Geometry check sheet. Reference: the model listing, model coordinates, mm. A direction names the side the tool comes from. Coordinates: 2 decimals unless noted, no trailing zeros. Order: outer loops, then holes, each group sorted by start corner. A loop starts at its lowest first (then second) coordinate and runs counter-clockwise, first axis right, second up. Notation, with made-up numbers: (1, 40) - (20, 40) arc R3 ccw to (20, 45) - close; hole circle Ø3 at (51.5, 21.25). An arc over 180 degrees is marked (long way). Put each result on its own line as item: value.
from build123d import *

# Parameters (mm, degrees)
SKETCH_1_R          = 42.5
SKETCH_1_R_2        = 35.25
EXTRUDE_1_DEPTH     = 2.5
SKETCH_2_R          = 1.5
CUT_EXTRUDE_1_DEPTH = 61.156047078
SKETCH_3_R          = 41.5
SKETCH_3_R_2        = 37.9
CUT_EXTRUDE_2_DEPTH = 0.5


with BuildPart() as part:
    # 草图1 → 凸台-拉伸1 (new body)
    with BuildSketch(Plane(origin=(0, 0, 0), x_dir=(1, 0, 0), z_dir=(0, 1, 0))):
        with Locations(Location((0, 0, 0), (0, 0, 270))):
            Circle(SKETCH_1_R)
        with Locations(Location((0, 0, 0), (0, 0, 270))):
            Circle(SKETCH_1_R_2, mode=Mode.SUBTRACT)
    extrude(amount=EXTRUDE_1_DEPTH)

    # 草图2 → 切除-拉伸1 (cut, through all)
    with BuildSketch(Plane.XZ):
        with Locations(Location((0, 40, 0), (0, 0, 270))):
            Circle(SKETCH_2_R)
        with Locations(Location((28.284271247, 28.284271247, 0), (0, 0, 270))):
            Circle(SKETCH_2_R)
        with Locations(Location((40, 0, 0), (0, 0, 270))):
            Circle(SKETCH_2_R)
        with Locations(Location((28.284271247, -28.284271247, 0), (0, 0, 270))):
            Circle(SKETCH_2_R)
        with Locations(Location((0, -40, 0), (0, 0, 270))):
            Circle(SKETCH_2_R)
        with Locations(Location((-28.284271247, -28.284271247, 0), (0, 0, 270))):
            Circle(SKETCH_2_R)
        with Locations(Location((-40, 0, 0), (0, 0, 270))):
            Circle(SKETCH_2_R)
        with Locations(Location((-28.284271247, 28.284271247, 0), (0, 0, 270))):
            Circle(SKETCH_2_R)
    extrude(amount=-CUT_EXTRUDE_1_DEPTH, mode=Mode.SUBTRACT)

    # 草图3 → 切除-拉伸2 (cut)
    with BuildSketch(Plane(origin=(0, 2.5, 0), x_dir=(1, 0, 0), z_dir=(0, 1, 0))):
        with Locations(Location((0, 0, 0), (0, 0, 270))):
            Circle(SKETCH_3_R)
        with Locations(Location((0, 0, 0), (0, 0, 270))):
            Circle(SKETCH_3_R_2, mode=Mode.SUBTRACT)
    extrude(amount=-CUT_EXTRUDE_2_DEPTH, mode=Mode.SUBTRACT)

    # 打孔尺寸(%根据十字)槽沉头木螺钉的类型1: read off the stored shape, not the designer's step
    # 打孔尺寸(%根据十字)槽沉头木螺钉的类型1: loft between two sections, ruled curve by curve
    hole_wizard_1_from = [
        Edge.make_three_point_arc((-40, 1.4, -1.5), (-38.5, 1.4, 0), (-40, 1.4, 1.5)),
        Edge.make_three_point_arc((-40, 1.4, 1.5), (-41.5, 1.4, 0), (-40, 1.4, -1.5)),
    ]
    hole_wizard_1_to = [
        Edge.make_three_point_arc((-40, -4.3e-08, -2.900000043), (-37.099999957, -4.3e-08, 0), (-40, -4.3e-08, 2.900000043)),
        Edge.make_three_point_arc((-40, -4.3e-08, 2.900000043), (-42.900000043, -4.3e-08, 0), (-40, -4.3e-08, -2.900000043)),
    ]
    hole_wizard_1 = Solid(Shell([*[Face.make_surface_from_curves(hole_wizard_1_from[k], hole_wizard_1_to[k]) for k in range(2)], Face(Wire(hole_wizard_1_from)), Face(Wire(hole_wizard_1_to))]))
    add(hole_wizard_1, mode=Mode.SUBTRACT)

    # Hole Wizard 1 2: loft between two sections, ruled curve by curve
    hole_wizard_1_2_from = [
        Edge.make_three_point_arc((-28.284271247, 1.4, -29.784271247), (-26.784271247, 1.4, -28.284271247), (-28.284271247, 1.4, -26.784271247)),
        Edge.make_three_point_arc((-28.284271247, 1.4, -26.784271247), (-29.784271247, 1.4, -28.284271247), (-28.284271247, 1.4, -29.784271247)),
    ]
    hole_wizard_1_2_to = [
        Edge.make_three_point_arc((-28.284271247, -4.3e-08, -31.18427129), (-25.384271205, -4.3e-08, -28.284271247), (-28.284271247, -4.3e-08, -25.384271205)),
        Edge.make_three_point_arc((-28.284271247, -4.3e-08, -25.384271205), (-31.18427129, -4.3e-08, -28.284271247), (-28.284271247, -4.3e-08, -31.18427129)),
    ]
    hole_wizard_1_2 = Solid(Shell([*[Face.make_surface_from_curves(hole_wizard_1_2_from[k], hole_wizard_1_2_to[k]) for k in range(2)], Face(Wire(hole_wizard_1_2_from)), Face(Wire(hole_wizard_1_2_to))]))
    add(hole_wizard_1_2, mode=Mode.SUBTRACT)

    # Hole Wizard 1 3: loft between two sections, ruled curve by curve
    hole_wizard_1_3_from = [
        Edge.make_three_point_arc((0, 1.4, -41.5), (1.5, 1.4, -40), (0, 1.4, -38.5)),
        Edge.make_three_point_arc((0, 1.4, -38.5), (-1.5, 1.4, -40), (0, 1.4, -41.5)),
    ]
    hole_wizard_1_3_to = [
        Edge.make_three_point_arc((0, -4.3e-08, -42.900000043), (2.900000043, -4.3e-08, -40), (0, -4.3e-08, -37.099999957)),
        Edge.make_three_point_arc((0, -4.3e-08, -37.099999957), (-2.900000043, -4.3e-08, -40), (0, -4.3e-08, -42.900000043)),
    ]
    hole_wizard_1_3 = Solid(Shell([*[Face.make_surface_from_curves(hole_wizard_1_3_from[k], hole_wizard_1_3_to[k]) for k in range(2)], Face(Wire(hole_wizard_1_3_from)), Face(Wire(hole_wizard_1_3_to))]))
    add(hole_wizard_1_3, mode=Mode.SUBTRACT)

    # Hole Wizard 1 4: loft between two sections, ruled curve by curve
    hole_wizard_1_4_from = [
        Edge.make_three_point_arc((28.284271247, 1.4, -29.784271247), (29.784271247, 1.4, -28.284271247), (28.284271247, 1.4, -26.784271247)),
        Edge.make_three_point_arc((28.284271247, 1.4, -26.784271247), (26.784271247, 1.4, -28.284271247), (28.284271247, 1.4, -29.784271247)),
    ]
    hole_wizard_1_4_to = [
        Edge.make_three_point_arc((28.284271247, -4.3e-08, -31.18427129), (31.18427129, -4.3e-08, -28.284271247), (28.284271247, -4.3e-08, -25.384271205)),
        Edge.make_three_point_arc((28.284271247, -4.3e-08, -25.384271205), (25.384271205, -4.3e-08, -28.284271247), (28.284271247, -4.3e-08, -31.18427129)),
    ]
    hole_wizard_1_4 = Solid(Shell([*[Face.make_surface_from_curves(hole_wizard_1_4_from[k], hole_wizard_1_4_to[k]) for k in range(2)], Face(Wire(hole_wizard_1_4_from)), Face(Wire(hole_wizard_1_4_to))]))
    add(hole_wizard_1_4, mode=Mode.SUBTRACT)

    # Hole Wizard 1 5: loft between two sections, ruled curve by curve
    hole_wizard_1_5_from = [
        Edge.make_three_point_arc((40, 1.4, -1.5), (41.5, 1.4, 0), (40, 1.4, 1.5)),
        Edge.make_three_point_arc((40, 1.4, 1.5), (38.5, 1.4, 0), (40, 1.4, -1.5)),
    ]
    hole_wizard_1_5_to = [
        Edge.make_three_point_arc((40, -4.3e-08, -2.900000043), (42.900000043, -4.3e-08, 0), (40, -4.3e-08, 2.900000043)),
        Edge.make_three_point_arc((40, -4.3e-08, 2.900000043), (37.099999957, -4.3e-08, 0), (40, -4.3e-08, -2.900000043)),
    ]
    hole_wizard_1_5 = Solid(Shell([*[Face.make_surface_from_curves(hole_wizard_1_5_from[k], hole_wizard_1_5_to[k]) for k in range(2)], Face(Wire(hole_wizard_1_5_from)), Face(Wire(hole_wizard_1_5_to))]))
    add(hole_wizard_1_5, mode=Mode.SUBTRACT)

    # Hole Wizard 1 6: loft between two sections, ruled curve by curve
    hole_wizard_1_6_from = [
        Edge.make_three_point_arc((28.284271247, 1.4, 26.784271247), (29.784271247, 1.4, 28.284271247), (28.284271247, 1.4, 29.784271247)),
        Edge.make_three_point_arc((28.284271247, 1.4, 29.784271247), (26.784271247, 1.4, 28.284271247), (28.284271247, 1.4, 26.784271247)),
    ]
    hole_wizard_1_6_to = [
        Edge.make_three_point_arc((28.284271247, -4.3e-08, 25.384271205), (31.18427129, -4.3e-08, 28.284271247), (28.284271247, -4.3e-08, 31.18427129)),
        Edge.make_three_point_arc((28.284271247, -4.3e-08, 31.18427129), (25.384271205, -4.3e-08, 28.284271247), (28.284271247, -4.3e-08, 25.384271205)),
    ]
    hole_wizard_1_6 = Solid(Shell([*[Face.make_surface_from_curves(hole_wizard_1_6_from[k], hole_wizard_1_6_to[k]) for k in range(2)], Face(Wire(hole_wizard_1_6_from)), Face(Wire(hole_wizard_1_6_to))]))
    add(hole_wizard_1_6, mode=Mode.SUBTRACT)

    # Hole Wizard 1 7: loft between two sections, ruled curve by curve
    hole_wizard_1_7_from = [
        Edge.make_three_point_arc((0, 1.4, 38.5), (1.5, 1.4, 40), (0, 1.4, 41.5)),
        Edge.make_three_point_arc((0, 1.4, 41.5), (-1.5, 1.4, 40), (0, 1.4, 38.5)),
    ]
    hole_wizard_1_7_to = [
        Edge.make_three_point_arc((0, -4.3e-08, 37.099999957), (2.900000043, -4.3e-08, 40), (0, -4.3e-08, 42.900000043)),
        Edge.make_three_point_arc((0, -4.3e-08, 42.900000043), (-2.900000043, -4.3e-08, 40), (0, -4.3e-08, 37.099999957)),
    ]
    hole_wizard_1_7 = Solid(Shell([*[Face.make_surface_from_curves(hole_wizard_1_7_from[k], hole_wizard_1_7_to[k]) for k in range(2)], Face(Wire(hole_wizard_1_7_from)), Face(Wire(hole_wizard_1_7_to))]))
    add(hole_wizard_1_7, mode=Mode.SUBTRACT)

    # Hole Wizard 1 8: loft between two sections, ruled curve by curve
    hole_wizard_1_8_from = [
        Edge.make_three_point_arc((-28.284271247, 1.4, 26.784271247), (-26.784271247, 1.4, 28.284271247), (-28.284271247, 1.4, 29.784271247)),
        Edge.make_three_point_arc((-28.284271247, 1.4, 29.784271247), (-29.784271247, 1.4, 28.284271247), (-28.284271247, 1.4, 26.784271247)),
    ]
    hole_wizard_1_8_to = [
        Edge.make_three_point_arc((-28.284271247, -4.3e-08, 25.384271205), (-25.384271205, -4.3e-08, 28.284271247), (-28.284271247, -4.3e-08, 31.18427129)),
        Edge.make_three_point_arc((-28.284271247, -4.3e-08, 31.18427129), (-31.18427129, -4.3e-08, 28.284271247), (-28.284271247, -4.3e-08, 25.384271205)),
    ]
    hole_wizard_1_8 = Solid(Shell([*[Face.make_surface_from_curves(hole_wizard_1_8_from[k], hole_wizard_1_8_to[k]) for k in range(2)], Face(Wire(hole_wizard_1_8_from)), Face(Wire(hole_wizard_1_8_to))]))
    add(hole_wizard_1_8, mode=Mode.SUBTRACT)


solid = part.part
Q1. Draft check along Z on faces 1 (the flat face through (35, 0, -6)), 2 (the cylindrical face through (12.465, 2.254, 39.584)), 3 (the cylindrical face through (-25.861, 1.232, -33.727)). Enter one of: pulls with the +Z half, pulls with the -Z half, needs draft (parallel to the pull), parting line crosses it, or undercut.
Answer block:
face 1: needs draft
face 2: undercut
face 3: parting line crosses it
Q2. Access from +Z, -Z, +X, -X, +Y, -Y to the whole of each face (thin tool, end or side, straight path). Record for faces 4 (the cylindrical face through (0.07, 1.7, 41.5)), 5 (the cylindrical face through (-36.999, 2.254, -8.216)).
Answer block:
face 4: +Y, -Y
face 5: +Y
Q3. Depth check by flat-ended pin: pin 1 Ø1.5 at (x, z) = (3.5, 33) entering from +Y; pin 2 Ø3.5 at (x, z) = (-40, 0) entering from -Y. Enter the tip coordinate at first touch or a pass-through.
Answer block:
pin 1: passes through
pin 2: stops at y = 1.15
Q4. Thickness scan on L1, parallel to X at y = 1.55, z = 0; L2, parallel to Z at x = 27, y = 1.4; L3, parallel to Z at x = -21, y = 2.1. Record the ranges inside material, lowest first. Write a range as [from, to].
Answer block:
L1: x = [-42.5, -41.5], [-38.5, -35.25], [35.25, 38.5], [41.5, 42.5]
L2: z = [-32.82, -29.06], [-27.51, -22.66], [22.66, 27.51], [29.06, 32.82]
L3: z = [-36.95, -35.79], [-31.55, -28.31], [28.31, 31.55], [35.79, 36.95]
Q5. Section check B-B on z = 20.5. Record the boundary of the cut face in (x, y), then the cut area to 3 significant figures.
Answer block:
outline: (-37.23, 0) - (-28.68, 0) - (-28.68, 2.5) - (-31.88, 2.5) - (-31.88, 2) - (-36.08, 2) - (-36.08, 2.5) - (-37.23, 2.5) - close; (28.68, 0) - (37.23, 0) - (37.23, 2.5) - (36.08, 2.5) - (36.08, 2) - (31.88, 2) - (31.88, 2.5) - (28.68, 2.5) - close
area: 38.6 mm^2
Q6. Section check A-A on x = 13. Record the boundary of the cut face in (y, z).
Answer block:
outline: (0, -40.46) - (2.5, -40.46) - (2.5, -39.41) - (2, -39.41) - (2, -35.6) - (2.5, -35.6) - (2.5, -32.77) - (0, -32.77) - close; (0, 32.77) - (2.5, 32.77) - (2.5, 35.6) - (2, 35.6) - (2, 39.41) - (2.5, 39.41) - (2.5, 40.46) - (0, 40.46) - close
